from build123d import *

# Parameters (mm, degrees)
SKETCH1_W               = 60
SKETCH1_H               = 40
BOSS_EXTRUDE1_DEPTH     = 5
CUT_EXTRUDE2_DEPTH      = 59.523499554
CUT_EXTRUDE2_DEPTH_BACK = 59.523499554
SKETCH2_W               = 1
SKETCH2_H               = 18.2
CUT_EXTRUDE3_DEPTH      = 7
SKETCH3_W               = 1
SKETCH3_H               = 18.2
CUT_EXTRUDE4_DEPTH      = 7
SKETCH6_W               = 40.00339764
SKETCH6_H               = 35.743622905
CUT_EXTRUDE5_DEPTH      = 7
SKETCH7_W               = 12.082118358
SKETCH7_H               = 49.934440021
CUT_EXTRUDE6_DEPTH      = 7


with BuildPart() as part:
    # Sketch1 → Boss-Extrude1 (new body)
    with BuildSketch(Plane.XY):
        with Locations((3.193565597, 28.20003109)):
            Rectangle(SKETCH1_W, SKETCH1_H)
    extrude(amount=BOSS_EXTRUDE1_DEPTH)

    # 3DSketch1 → Cut-Extrude2 (cut, two sides)
    with BuildSketch(Plane(origin=(-16.806434403, 18.20003109, 5), x_dir=(0.8944271909999159, 0.4472135954999582, 0), z_dir=(0, 0, 1))) as cut_extrude2_sk:
        Polygon((0, 0), (35.77708764, -17.88854382), (44.72135955, 0), (8.94427191, 17.88854382), align=None)
    extrude(amount=CUT_EXTRUDE2_DEPTH, mode=Mode.SUBTRACT)
    extrude(cut_extrude2_sk.sketch, amount=-CUT_EXTRUDE2_DEPTH_BACK, mode=Mode.SUBTRACT)

    # Sketch2 → Cut-Extrude3 (cut)
    with BuildSketch(Plane(origin=(-16.806434403, 0, 0), x_dir=(0, 0, -1), z_dir=(1, 0, 0))):
        with Locations((-3.8, 28.20003109)):
            Rectangle(SKETCH2_W, SKETCH2_H)
    extrude(amount=-CUT_EXTRUDE3_DEPTH, mode=Mode.SUBTRACT)

    # Sketch3 → Cut-Extrude4 (cut)
    with BuildSketch(Plane.ZY.offset(-23.193565597)):
        with Locations((3.8, 28.20003109)):
            Rectangle(SKETCH3_W, SKETCH3_H)
    extrude(amount=-CUT_EXTRUDE4_DEPTH, mode=Mode.SUBTRACT)

    # Sketch6 → Cut-Extrude5 (cut)
    with BuildSketch(Plane.XY.offset(5)):
        with Locations((3.195264417, 28.798257348)):
            Rectangle(SKETCH6_W, SKETCH6_H)
    extrude(amount=-CUT_EXTRUDE5_DEPTH, mode=Mode.SUBTRACT)

    # Sketch7 → Cut-Extrude6 (cut)
    with BuildSketch(Plane.XY.offset(5)):
        with Locations((35.534916951, 27.405939639)):
            Rectangle(SKETCH7_W, SKETCH7_H)
    extrude(amount=-CUT_EXTRUDE6_DEPTH, mode=Mode.SUBTRACT)


solid = part.part
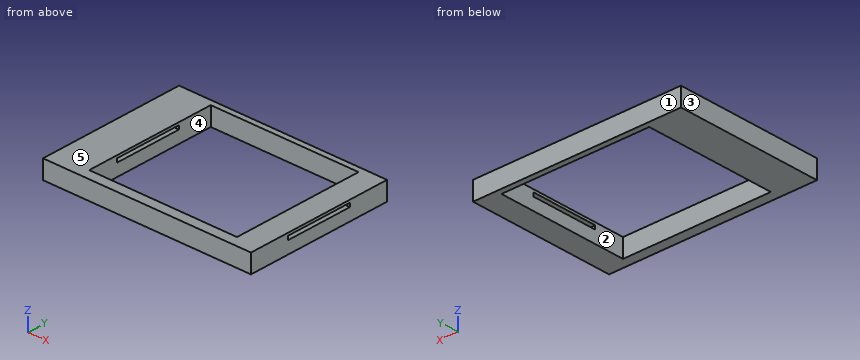
Model file for the job. Use its own axes, mm. Face numbers are marked on the shaded views. A direction names the side the tool comes from. Round coordinates to 2 decimals unless told otherwise and drop trailing zeros. Loops run counter-clockwise (first coordinate to the right, second up) from the corner with the lowest first, then second, coordinate; pieces in that order, holes last. Notation, with made-up numbers: (47, 64.5) -> (57, 64.5) arc R14 cw to (57, 74.5) -> close; hole circle Ø9 at (44.25, -14). An arc over 180 degrees is marked (long way). Answer as CSV lines item,"result". Start each with the question number.
1) Slice it at C-C (z = 1.1). List the corners of the cut face in (x, y), plus the area to 3 significant figures.
2) Probe line 1 along Y through (x, z) = (5, 1.9); line 2 along Z through (x, y) = (27, 26); line 3 along X through (y, z) = (27.5, 0.75). List the from-to ranges inside material, lowest first.
3) Slice it at A-A (y = 13). List the corners of the cut face in (x, z), plus the area to 3 significant figures.
4) Slice it at D-D (x = -21). List the corners of the cut face in (y, z).
5) Mould opens along X. For the marked faces 1, 2 and 3 say: +X half, -X half, draft (parallel to the pull), parting line (faces both ways), or undercut.
6) Tool access for the marked faces 4 and 5: list every direction of +Z, -Z, +X, -X, +Y, -Y with a clear straight run to the whole face (end or side of a thin tool).
7) Pin check, flat tips, straight feed: P1, Ø1.5, axis at x = -15, y = 25, coming from the -Z side; P2, Ø0.5, axis at y = 25, z = 4, coming from the +X side. Stop position of each tip, or through.
8) Slice it at B-B (x = -4). List the corners of the cut face in (y, z).
Filled in:
1,outline,"(-26.81, 8.2) -> (29.49, 8.2) -> (29.49, 48.2) -> (-26.81, 48.2) -> close; hole (-16.81, 10.93) -> (23.2, 10.93) -> (23.2, 46.67) -> (-16.81, 46.67) -> close"
1,area,"822 mm2"
2,line 1,"y = 8.2 to 10.93, 46.67 to 48.2"
2,line 2,"z = 0 to 3.3, 4.3 to 5"
2,line 3,"x = -26.81 to -16.81, 23.2 to 29.49"
3,outline,"(-26.81, 0) -> (-16.81, 0) -> (-16.81, 5) -> (-26.81, 5) -> close; (23.2, 0) -> (29.49, 0) -> (29.49, 5) -> (23.2, 5) -> close"
3,area,"81.5 mm2"
4,outline,"(8.2, 0) -> (48.2, 0) -> (48.2, 5) -> (8.2, 5) -> close; hole (19.1, 3.3) -> (37.3, 3.3) -> (37.3, 4.3) -> (19.1, 4.3) -> close"
5,face 1,"draft"
5,face 2,"undercut"
5,face 3,"-X half"
6,face 4,"+Z, -Z"
6,face 5,"+Z, +X, -X, +Y, -Y"
7,P1,"passes through"
7,P2,"stops at x = -23.81"
8,outline,"(8.2, 0) -> (10.93, 0) -> (10.93, 5) -> (8.2, 5) -> close; (46.67, 0) -> (48.2, 0) -> (48.2, 5) -> (46.67, 5) -> close"
